Geometry: final body of the model. Coordinates: model frame, mm. A direction names the side the tool comes from. Give positions to 0.01 mm unless a question says otherwise; leave off trailing zeros. Loops run counter-clockwise (first coordinate to the right, second up) from the corner with the lowest first, then second, coordinate; pieces in that order, holes last. Notation, with made-up numbers: (27.25, -28.5) -> (33.25, -28.5) arc R38 ccw to (33.25, 9.5) -> close; hole circle Ø2 at (53.25, 10). An arc over 180 degrees is marked (long way). One line per question, with ' | ' between items. Start each with the question number.
Item 1: Set-up query: faces 5 (the cylindrical face through (0, 2, 3)), 6 (the flat face through (0, 0, 0)), 7 (the flat face through (0, 0, 7)). Return all of +Z, -Z, +X, -X, +Y, -Y with unobstructed straight access to the full face (end or side cutting, diameter ignored); none if empty.
Item 2: Material intervals for line 1 along Z through (x, y) = (0, 0.5); line 2 along Y through (x, z) = (-0.25, 8.75); line 3 along Y through (x, z) = (-3.5, 6.5), sorted ascending. Write a range as [from, to].
Item 3: Mould query, pull axis X, two halves, no side actions, for faces 1 (the flat face through (-0.616, -1.088, 8.014)), 2 (the cylindrical face through (-0.867, 3.905, 6.246)), 3 (the flat face through (0.63, -1.08, 8.01)), 4 (the flat face through (-2, -1, 6)). Classes: released by +X, released by -X, zero draft, split by the parting line, or undercut.
Item 4: Section A-A on z = 3.75. Return loops of the section in (x, y).
Item 5: Pin query (flat end, axial travel): P1, Ø1.6, axis at y = -0.5, z = 8.5, coming from the -X side; P2, Ø0.8, axis at x = -0.5, y = 0, coming from the +Z side; P3, Ø1.5, axis at x = -0.5, z = 3.5, coming from the -Y side. Return the tip coordinate at first contact, or that it passes through.
Autodesk Inventor part; units mm, degrees
ref_plane "YZ Plane" through (0, 0, 0) normal (1, 0, 0) x (0, 1, 0)
ref_plane "XZ Plane" through (0, 0, 0) normal (0, 1, 0) x (-1, 0, 0)
ref_plane "XY Plane" through (0, 0, 0) normal (0, 0, 1) x (1, 0, 0)
sketch "スケッチ1" plane through (0, 0, 0) normal (0, 0, 1) x (1, 0, 0)
  circle A0 centre (0, 0) radius 2
  dimension "d0" = 4
extrude "押し出し1" add sketch "スケッチ1" along normal blind 6
sketch "スケッチ2" plane through (0, 0, 6) normal (0, 0, 1) x (1, 0, 0)
  circle A0 centre (0, 0) radius 2
  circle A1 centre (0, 0) radius 4
  dimension "d3" = 8
extrude "押し出し2" add sketch "スケッチ2" along normal blind 3 contours A0 | A1
fillet "フィレット1" radius 2.5 1 edges at (-4, 0, 9)
thread "ねじ1"
sketch "スケッチ3" plane through (0, 0, 9) normal (0, 0, 1) x (1, 0, 0)
  line L0 (0, 1.4434) -> (1.25, 0.7217)
  line L1 (1.25, 0.7217) -> (1.25, -0.7217)
  line L2 (1.25, -0.7217) -> (0, -1.4434)
  line L3 (0, -1.4434) -> (-1.25, -0.7217)
  line L4 (-1.25, -0.7217) -> (-1.25, 0.7217)
  line L5 (-1.25, 0.7217) -> (0, 1.4434)
  point P0 (0, 0)
  point P1 (0, 0)
  dimension "d10" = 2.5
extrude "押し出し3" cut sketch "スケッチ3" against normal blind 2
properties part number "ネジボタン4L6" material "Stainless Steel, 440C"
Result sheet:
1) face 5: -Z | face 6: -Z, +X, -X, +Y, -Y | face 7: +Z
2) line 1: z = [0, 7] | line 2: y = [-2.58, -1.3], [1.3, 2.58] | line 3: y = [-1.94, 1.94]
3) face 1: undercut | face 2: split by the parting line | face 3: undercut | face 4: zero draft
4) outline: circle Ø4 at (0, 0)
5) P1: stops at x = -3.67 | P2: stops at z = 7 | P3: stops at y = -2
